```python
from build123d import *

# Parameters (mm, degrees)
F0_R     = 12.7
F1_DEPTH = 50.8
F3_D     = 19.05
F3_DEPTH = 25.4
F3_TIP   = 5.7231973962


# Not quite as in the source:
# - a fillet or chamfer that OpenCascade refuses, or shapes differently, is made with other operations: its cross-section is extruded or revolved along the edge and cut away or added


with BuildPart() as f1:
    # F0 (on Top) → F1 (new body)
    with BuildSketch(Plane.XY):
        Circle(F0_R)
    extrude(amount=F1_DEPTH)

    # F3
    with Locations(Plane(origin=(0, 0, 0), x_dir=(1, 0, 0), z_dir=(0, 0, -1))):
        with Locations((0, 0)):
            Hole(F3_D / 2, depth=F3_DEPTH)
            with Locations((0, 0, -(F3_DEPTH + F3_TIP / 2))):  # 118° drill point
                Cone(0, F3_D / 2, F3_TIP, mode=Mode.SUBTRACT)

    # F4: fillet of radius 5.08 on 1 edges, made by hand

    # F4_s1 → F4_t2 (revolve, cut)
    with BuildSketch(Plane.XZ):
        with BuildLine():
            ThreePointArc((12.7, 4.7092860393), (11.8321134838, 1.8694797079), (9.525, 0))
            Line((9.525, 0), (12.7, 0))
            Line((12.7, 0), (12.7, 4.7092860393))
        make_face()
    revolve(axis=Axis((0, 0, 0), (0, 0, 1)), mode=Mode.SUBTRACT)


solid = f1.part
```
Source: CAD feature listing. Evaluate the final solid. Frame: model axes, mm. Coordinates: 2 decimals unless noted, no trailing zeros. Write each loop counter-clockwise with the first axis right and the second up, starting at its lowest first coordinate (ties: lowest second). Pieces come first, ordered by that corner, then holes. Notation, with made-up numbers: (-33, 82.25) - (-29, 82.25) arc R24 ccw to (-29, 95.25) - close; hole circle Ø2 at (2.5, 25). An arc over 180 degrees is marked (long way). Answer as a JSON object with one key per item and string values.
Q1. Draft query along X for faces 1 (the cylindrical face through (-2.75, -12.4, 27.43)), 2 (the cylindrical face through (7.559, 5.796, 12.878)), 3 (the flat face through (0, 0, 50.8)). Return one class per face: released by +X, released by -X, zero draft, split by the parting line, or undercut.
Ans:
{"face 1": "split by the parting line", "face 2": "undercut", "face 3": "zero draft"}
Q2. Material intervals for line 1 (Y direction, x = 0, z = 15.75) (3 decimals); line 2 (Y direction, x = -1, z = 30); line 3 (X direction, y = -1.75, z = 17.5), sorted ascending. Write a range as [from, to].
Ans:
{"line 1": "y = [-12.7, -9.525], [9.525, 12.7]", "line 2": "y = [-12.66, -1.58], [1.58, 12.66]", "line 3": "x = [-12.58, -9.36], [9.36, 12.58]"}
Q3. Section query A-A, the plane z = 19. Output: boundary loops of the cut face in (x, y) (3 decimals), plus the area to 3 significant figures.
Ans:
{"outline": "circle Ø25.4 at (0, 0); hole circle Ø19.05 at (0, 0)", "area": "222 mm2"}
Q4. Section query B-B, the plane z = 47. Output: boundary loops of the cut face in (x, y), plus the area to 3 significant figures.
Ans:
{"outline": "circle Ø25.4 at (0, 0)", "area": "507 mm2"}
Q5. First-contact query: pin 1 Ø3 at (x, z) = (8, 43) entering from +Y; pin 2 Ø12 at (y, z) = (-8.5, 20) entering from +X; pin 3 Ø2 at (x, z) = (-1.5, 12) entering from +Y. Flat tips, straight axial feed; report the tip coordinate or a pass-through.
Ans:
{"pin 1": "stops at y = 10.91", "pin 2": "stops at x = 12.45", "pin 3": "stops at y = 12.69"}
